Verification items for the finished model (mm, model axes). Face numbers are marked on the shaded views. A direction names the side the tool comes from. Coordinates: 2 decimals unless noted, no trailing zeros. Write each loop counter-clockwise with the first axis right and the second up, starting at its lowest first coordinate (ties: lowest second). Pieces come first, ordered by that corner, then holes. Notation, with made-up numbers: (40.25, -20.5) -> (85.25, -20.5) arc R27 ccw to (85.25, 16.5) -> close; hole circle Ø4 at (68.25, 62.25). An arc over 180 degrees is marked (long way). Answer in a Markdown table with one row per item.
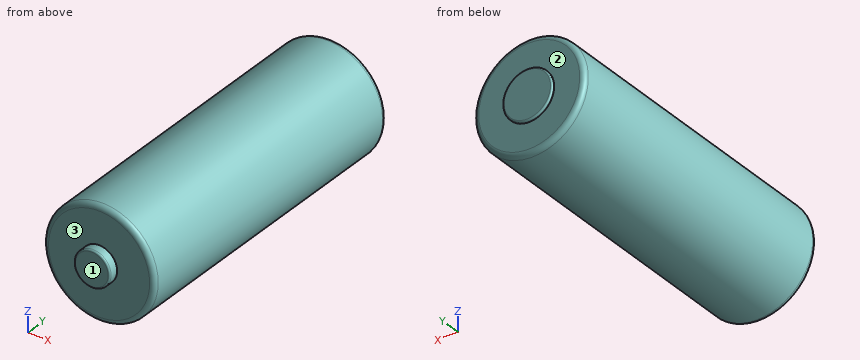
```python
from build123d import *

# Parameters (mm, degrees)
F0_R     = 8.4963
F1_DEPTH = 48.768
F2_R     = 2.7559
F3_DEPTH = 1.524
F4_R     = 3.81
F5_DEPTH = 0.4064
F6_R     = 0.254
F7_R     = 0.762


with BuildPart() as f1:
    # F0 (on Front) → F1 (new body)
    with BuildSketch(Plane.XZ):
        Circle(F0_R)
    extrude(amount=-F1_DEPTH)

    # F2 (on face) → F3 (join)
    with BuildSketch(Plane.XZ):
        Circle(F2_R)
    extrude(amount=F3_DEPTH)

    # F4 (on face) → F5 (join)
    with BuildSketch(Plane(origin=(0, 48.768, 0), x_dir=(-1, 0, 0), z_dir=(0, 1, 0))):
        Circle(F4_R)
    extrude(amount=F5_DEPTH)

    # F6
    f6_edges = [f1.edges().sort_by_distance(p)[0] for p in [
        (3.81, 49.1744, 0),
        (-2.7559, -1.524, 0),
    ]]
    fillet(f6_edges, radius=F6_R)

    # F7
    f7_edges = [f1.edges().sort_by_distance(p)[0] for p in [
        (-8.4963, 48.768, 0),
        (-8.4963, 0, 0),
    ]]
    fillet(f7_edges, radius=F7_R)


solid = f1.part
```
1. Section check C-C, the plane y = 15. Record the boundary of the cut face in (x, z).
Geometry says:
| item | result |
|---|---|
| outline | circle Ø16.99 at (0, 0) |
2. Section check B-B, the plane z = 0. Record the boundary of the cut face in (x, y), plus the area to 3 significant figures.
Geometry says:
| item | result |
|---|---|
| outline | (-8.5, 0.76) arc R0.76 ccw to (-7.73, 0) -> (-2.76, 0) -> (-2.76, -1.27) arc R0.25 ccw to (-2.5, -1.52) -> (2.5, -1.52) arc R0.25 ccw to (2.76, -1.27) -> (2.76, 0) -> (7.73, 0) arc R0.76 ccw to (8.5, 0.76) -> (8.5, 48.01) arc R0.76 ccw to (7.73, 48.77) -> (3.81, 48.77) -> (3.81, 48.92) arc R0.25 ccw to (3.56, 49.17) -> (-3.56, 49.17) arc R0.25 ccw to (-3.81, 48.92) -> (-3.81, 48.77) -> (-7.73, 48.77) arc R0.76 ccw to (-8.5, 48.01) -> close |
| area | 840 mm^2 |
3. Thickness scan on line 1 (Y direction, x = -0.25, z = 6.5); line 2 (X direction, y = 36, z = 0.25); line 3 (Z direction, x = -3.5, y = 44). Record the ranges inside material, lowest first. Write a range as from..to.
Geometry says:
| item | result |
|---|---|
| line 1 | 0..48.77 |
| line 2 | -8.49..8.49 |
| line 3 | -7.74..7.74 |
4. Depth check by flat-ended pin: P1, Ø1.5, axis at y = 37.5, z = 3.5, coming from the -X side; P2, Ø2, axis at x = 3.5, y = 38.5, coming from the -Z side; P3, Ø4, axis at x = -6, y = 25.5, coming from the +Z side; P4, Ø4.5, axis at x = 1, z = 3.5, coming from the -Y side. Enter the tip coordinate at first touch or a pass-through.
Geometry says:
| item | result |
|---|---|
| P1 | x = -8.04 |
| P2 | z = -8.12 |
| P3 | z = 7.5 |
| P4 | y = -1.52 |
5. Tool access check on the marked faces 1, 2 and 3. Record the directions out of +Z, -Z, +X, -X, +Y, -Y that give a thin tool (end or side, any length) a straight path to the whole face; none if there is none.
Geometry says:
| item | result |
|---|---|
| face 1 | +Z, -Z, +X, -X, -Y |
| face 2 | +Y |
| face 3 | -Y |
6. Section check A-A, the plane x = 0. Record the boundary of the cut face in (y, z).
Geometry says:
| item | result |
|---|---|
| outline | (-1.52, -2.5) arc R0.25 ccw to (-1.27, -2.76) -> (0, -2.76) -> (0, -7.73) arc R0.76 ccw to (0.76, -8.5) -> (48.01, -8.5) arc R0.76 ccw to (48.77, -7.73) -> (48.77, -3.81) -> (48.92, -3.81) arc R0.25 ccw to (49.17, -3.56) -> (49.17, 3.56) arc R0.25 ccw to (48.92, 3.81) -> (48.77, 3.81) -> (48.77, 7.73) arc R0.76 ccw to (48.01, 8.5) -> (0.76, 8.5) arc R0.76 ccw to (0, 7.73) -> (0, 2.76) -> (-1.27, 2.76) arc R0.25 ccw to (-1.52, 2.5) -> close |
